Here's how the part is built. I have some questions about the finished solid (model axes, mm). A direction names the side the tool comes from. Round coordinates to 2 decimals unless told otherwise and drop trailing zeros. Loops run counter-clockwise (first coordinate to the right, second up) from the corner with the lowest first, then second, coordinate; pieces in that order, holes last. Notation, with made-up numbers: M 32.25,82 L 81.25,82 A16 cw 81.25,92 Z; hole C 57,18 d5. An arc over 180 degrees is marked long. Answer as a JSON object with one key per item and string values.
from build123d import *

# Parameters (mm, degrees)
PAD007_DEPTH         = 12
SKETCH065_R          = 2.2
POCKET021_DEPTH      = 0.001
POCKET021_DEPTH_BACK = 42.001
SKETCH025_R          = 1.65
POCKET022_DEPTH      = 9.638709
POCKET022_DEPTH_BACK = 9.638709


with BuildPart() as part:
    # Sketch023 → Pad007 (new body)
    with BuildSketch(Plane.YZ):
        Polygon((42, 42), (42, 30), (19.75, 30), (-19.75, 30), (-42, 30), (-42, 42), (-11, 42), (11, 42), align=None)
    extrude(amount=PAD007_DEPTH)

    # Sketch065 → Pocket021 (cut, two sides)
    with BuildSketch(Plane.XY) as pocket021_sk:
        with Locations((6, 30.875)):
            Circle(SKETCH065_R)
        with Locations((6, -30.875)):
            Circle(SKETCH065_R)
        Polygon((10.866975, 6.950634), (13, 9.083659), (13, -5.999897), (12, -5.999897), align=None)
        Polygon((0, 5.999897), (-1, 5.999897), (-1, -9.083659), (1.133025, -6.950634), align=None)
    extrude(amount=-POCKET021_DEPTH, mode=Mode.SUBTRACT)
    extrude(pocket021_sk.sketch, amount=POCKET021_DEPTH_BACK, mode=Mode.SUBTRACT)

    # Sketch025 (on DatumPlane) → Pocket022 (cut, two sides)
    with BuildSketch(Plane(origin=(6, 0, 0), x_dir=(-0.087156, 0.996195, 0), z_dir=(0.996195, 0.087156, 0))) as pocket022_sk:
        with Locations((0, 33)):
            Circle(SKETCH025_R)
    extrude(amount=-POCKET022_DEPTH, mode=Mode.SUBTRACT)
    extrude(pocket022_sk.sketch, amount=POCKET022_DEPTH_BACK, mode=Mode.SUBTRACT)


with BuildPart() as part_1:
    # Body008 placement: moved
    add(part.part.moved(Location((122.7, 0, 834))))


solid = part_1.part
Item 1: We'd pull the mould along Y, two halves only. Please class faces 4 (the face through (134.7, 25, 870)), 5 (the face through (129, -42, 870)), 6 (the face through (128.88, -1.2, 868.12)): +Y half, -Y half, draft (parallel to the pull), parting line (faces both ways), or undercut.
Solution:
{"face 4": "draft", "face 5": "-Y half", "face 6": "undercut"}
Item 2: I want a section at A-A on z = 867.75. List the corners of the cut face in (x, y) for me (3 decimals), plus the area to 3 significant figures.
Solution:
{"outline": "M 122.7,-42 L 134.7,-42 L 134.7,-6 L 134.262,-0.989 L 123.395,-1.939 L 123.833,-6.951 L 122.7,-8.084 Z; M 122.7,6 L 123.138,0.989 L 134.005,1.939 L 133.567,6.951 L 134.7,8.084 L 134.7,42 L 122.7,42 Z; hole C 128.7,-30.875 d4.4; hole C 128.7,30.875 d4.4", "area": "930 mm2"}
Item 3: For faces 1 (the face through (122.7, 24, 870)), 2 (the face through (134.14, 0.38, 869.92)), 3 (the face through (123.274, -0.566, 869.916)), which set-ups out of +Z, -Z, +X, -X, +Y, -Y let a thin tool reach every point of the face, with its end or its side?
Solution:
{"face 1": "+Z, -Z, -X, +Y, -Y", "face 2": "+Z, -Z, +X", "face 3": "+Z, -Z, -X"}
Item 4: I want a section at B-B on z = 875.25. List the corners of the cut face in (x, y) for me (3 decimals), plus the area to 3 significant figures.
Solution:
{"outline": "M 122.7,-42 L 134.7,-42 L 134.7,-6 L 133.567,6.951 L 134.7,8.084 L 134.7,42 L 122.7,42 L 122.7,6 L 123.833,-6.951 L 122.7,-8.084 Z; hole C 128.7,-30.875 d4.4; hole C 128.7,30.875 d4.4", "area": "962 mm2"}
Item 5: I want a section at C-C on y = -30. List the corners of the cut face in (x, z) for me.
Solution:
{"outline": "M 122.7,864 L 126.68,864 L 126.68,876 L 122.7,876 Z; M 130.72,864 L 134.7,864 L 134.7,876 L 130.72,876 Z"}
Item 6: If I drill on L1, parallel to Y at x = 128.7, z = 871.25 (3 decimals); L2, parallel to Y at x = 126.75, z = 866.5; L3, parallel to Y at x = 128.5, z = 867.25, over which ranges is the centre line in solid material (lowest first)? Write a range as from..to.
Solution:
{"L1": "y = -42..-33.075, -28.675..28.675, 33.075..42", "L2": "y = -42..-31.89, -29.86..-1.75, 1.41..29.86, 31.89..42", "L3": "y = -42..-33.07, -28.68..-1.65, 1.62..28.68, 33.07..42"}
Item 7: I want a section at D-D on x = 129. Count the separate pieces of the cut face and the enclosed holes in it, plus the area to 3 significant figures.
Solution:
{"separate pieces": "3", "enclosed holes": "1", "area": "895 mm2"}
